Build history of the part. All positions in model axes, mm. Face numbers are marked on the shaded views. A direction names the side the tool comes from. Round coordinates to 2 decimals unless told otherwise and drop trailing zeros. Write each loop counter-clockwise with the first axis right and the second up, starting at its lowest first coordinate (ties: lowest second). Pieces come first, ordered by that corner, then holes.
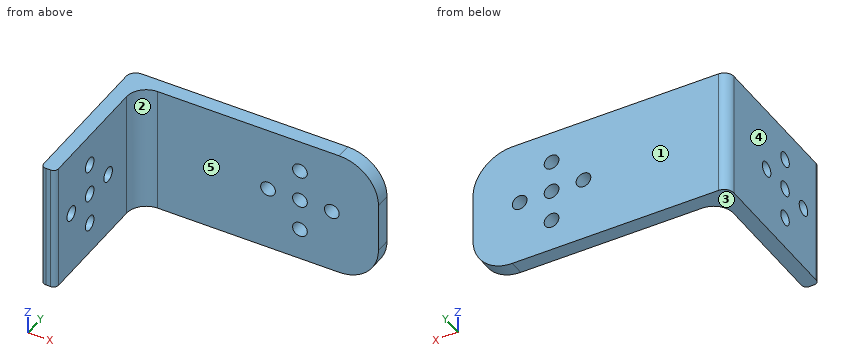
Autodesk Inventor part; units mm, degrees
ref_plane "YZ Plane" through (0, 0, 0) normal (1, 0, 0) x (0, 1, 0)
ref_plane "XZ Plane" through (0, 0, 0) normal (0, 1, 0) x (-1, 0, 0)
ref_plane "XY Plane" through (0, 0, 0) normal (0, 0, 1) x (1, 0, 0)
sketch "Sketch1" plane through (0, 0, 0) normal (0, 0, 1) x (1, 0, 0)
  line L0 (0, 0) -> (-49, 0)
  line L1 (-49, 0) -> (-49, 18)
  line L2 (-49, 18) -> (0, 18) construction
  line L3 (-49, 18) -> (-52, 18)
  line L4 (-52, 18) -> (-52, -3)
  line L5 (-52, -3) -> (0, -3)
  line L6 (0, -3) -> (0, 0)
  dimension "d0" = 18
  dimension "d1" = 3
  dimension "d2" = 3
  dimension "d3" = 52
extrude "Extrusion1" add sketch "Sketch1" along normal blind 10
mirror "Mirror1" about plane through (-32.0411, 1.4589, 0) normal (0, 0, -1) of "Extrusion1"
mirror "Mirror2" about plane through (-49, 18, 0) normal (0, 1, 0) of "Extrusion1", "Mirror1"
sketch "Sketch4" plane through (0, -3, -10) normal (0, 0, -1) x (-1, 0, 0)
  line L0 (0, 3) -> (49, 3)
  line L1 (0, 0) -> (0, 3)
  line L2 (52, 0) -> (0, 0)
  line L3 (52, 42) -> (52, 0)
  line L4 (52, 42) -> (0, 42)
  line L5 (0, 42) -> (0, 39)
  line L6 (0, 39) -> (49, 39)
  line L7 (49, 39) -> (49, 3)
  line L8 (0, 3) -> (49, 3)
  line L9 (0, 0) -> (0, 3)
  line L10 (52, 0) -> (0, 0)
  line L11 (52, 42) -> (52, 0)
  line L12 (52, 42) -> (0, 42)
  line L13 (0, 42) -> (0, 39)
  line L14 (0, 39) -> (49, 39)
  line L15 (49, 39) -> (49, 3)
extrude "Extrusion4" add sketch "Sketch4" along normal blind 5
mirror "Mirror3" about plane through (0, 0, 0) normal (0, 0, 1) of "Extrusion4"
sketch "Sketch11" plane through (-52, -3, -15) normal (0, -1, 0) x (1, 0, 0)
  line L0 (52, 0) -> (52, 30)
  line L1 (52, 30) -> (0, 30)
  line L2 (0, 0) -> (0, 30)
  line L3 (52, 0) -> (0, 0)
  line L4 (52, 0) -> (52, 30)
  line L5 (52, 30) -> (0, 30)
  line L6 (0, 0) -> (0, 30)
  line L7 (52, 0) -> (0, 0)
  point P0 (52, 15)
extrude "Extrusion11" cut sketch "Sketch11" against normal blind 10
sketch "Sketch13" plane through (0, 36, -15) normal (1, 0, 0) x (0, 0, -1)
  line L0 (-30, 3) -> (-28, 3)
  line L1 (-28, 3) -> (-28, -29)
  line L2 (-28, -29) -> (-30, -29)
  line L3 (-30, -29) -> (-30, 3)
  line L4 (-30, -29) -> (0, -29)
  point P0 (-15, -36)
  dimension "d65" = 2
extrude "Extrusion13" cut sketch "Sketch13" against normal up to next
mirror "Mirror4" about plane through (0, 0, 0) normal (0, 0, 1) of "Extrusion13"
sketch "Sketch14" plane through (-52, 7, 13) normal (-1, 0, 0) x (0, 0, 1)
  line L0 (-26, 32) -> (-26, 0)
  line L1 (-26, 0) -> (0, 0)
  line L2 (0, 32) -> (-26, 32)
  circle A0 centre (-13, 12) radius 6.5 construction
  line L3 (-13, 12) -> (-26, 12) construction
  line L4 (-13, 12) -> (-13, 32) construction
  circle A1 centre (-13, 12) radius 1.5
  circle A2 centre (-13, 18.5) radius 1.5
  point P0 (-13, -7)
  point P1 (-13, 0)
  dimension "d68" = 13
  dimension "d69" = 20
  dimension "d71" = 3
  dimension "d72" = 3
extrude "Extrusion14" cut sketch "Sketch14" against normal up to next
pattern_circular "Circular Pattern6" count 4 over 360 about axis through (-52, 19, 0) along (1, 0, 0) of "Extrusion14"
sketch "Sketch15" plane through (-49, 36, 13) normal (0, -1, 0) x (1, 0, 0)
  line L0 (49, -26) -> (49, 0)
  line L1 (49, 0) -> (0, 0)
  circle A0 centre (33, -13) radius 6.5 construction
  line L2 (33, -13) -> (33, 0) construction
  circle A1 centre (33, -6.5) radius 1.5
  circle A2 centre (33, -13) radius 1.5
  point P0 (49, -13)
  point P1 (49, -13)
  dimension "d78" = 13
  dimension "d79" = 16
  dimension "d80" = 3
  dimension "d81" = 3
extrude "Extrusion15" cut sketch "Sketch15" against normal up to next
pattern_circular "Circular Pattern7" count 4 over 360 about axis through (-16, 36, 0) along (0, 1, 0) of "Extrusion15"
fillet "Fillet1" radius 8 2 edges at (0, 37.5, -13) (0, 37.5, 13)
sketch "Sketch18" plane through (-52, 39, 13) normal (0, 1, 0) x (1, 0, 0)
  arc A0 (44, 0) -> (52, 8) centre (44, 8) ccw
  line L0 (52, 8) -> (52, 18)
  arc A1 (52, 18) -> (44, 26) centre (44, 18) ccw
  line L1 (44, 26) -> (0, 26)
  line L2 (0, 0) -> (0, 26)
  line L3 (0, 0) -> (44, 0)
  circle A2 centre (36, 13) radius 1.5
  circle A3 centre (36, 6.5) radius 1.5
  circle A4 centre (29.5, 13) radius 1.5
  circle A5 centre (42.5, 13) radius 1.5
  circle A6 centre (36, 19.5) radius 1.5
  point P0 (52, 13)
  dimension "d93" = 26
fillet "Fillet2" radius 4 1 edges at (-49, 36, 0)
fillet "Fillet3" radius 2 1 edges at (-52, 39, 0)
fillet "Fillet4" radius 1 2 edges at (-49, 7, 0) (-52, 7, 0)
equation "\"d72\" = d71"
properties part number "L_micro_sergei_dines"
1) Pin check, flat tips, straight feed: pin 1 Ø2.5 at (y, z) = (25.5, 0) entering from -X; pin 2 Ø3.5 at (y, z) = (12.5, 0) entering from -X; pin 3 Ø8 at (x, z) = (-22, 5.5) entering from -Y; pin 4 Ø12 at (y, z) = (20, 2.5) entering from +X. Stop position of each tip, or through.
Results:
pin 1: passes through
pin 2: stops at x = -52
pin 3: stops at y = 36
pin 4: stops at x = -49
2) Which spindle directions (+Z, -Z, +X, -X, +Y, -Y) get a long thin tool onto all of the face, cutting with end or side? Do the marked faces 4 and 5. Say none if no direction does.
Results:
face 4: +Z, -Z, -X, +Y, -Y
face 5: +Z, -Z, +X, -Y
3) Wall check: L1, parallel to Y at x = -14.5, z = 1.5; L2, parallel to X at y = 13, z = 6; L3, parallel to Z at x = -22.5, y = 37.9. Give the ranges that are in metal, low to high.
Results:
L1: y = 36 to 39
L2: x = -52 to -49
L3: z = -13 to -1.5, 1.5 to 13
4) Slice it at A-A (y = 19). Write the cut outline in (x, z).
Results:
outline: (-52, -13) - (-49, -13) - (-49, -8) - (-52, -8) - close; (-52, -5) - (-49, -5) - (-49, -1.5) - (-52, -1.5) - close; (-52, 1.5) - (-49, 1.5) - (-49, 5) - (-52, 5) - close; (-52, 8) - (-49, 8) - (-49, 13) - (-52, 13) - close
5) Mould opens along Y. For the marked faces 1, 2 and 3 say: released by +Y, released by -Y, zero draft, split by the parting line, or undercut.
Results:
face 1: released by +Y
face 2: released by -Y
face 3: zero draft
6) Slice it at D-D (y = 25.5). Write the cut outline in (x, z), plus the area to 3 significant figures.
Results:
outline: (-52, -13) - (-49, -13) - (-49, -1.5) - (-52, -1.5) - close; (-52, 1.5) - (-49, 1.5) - (-49, 13) - (-52, 13) - close
area: 69.0 mm2
7) Slice it at C-C (x = -22.5). Write the cut outline in (y, z), plus the area to 3 significant figures.
Results:
outline: (36, -13) - (39, -13) - (39, -1.5) - (36, -1.5) - close; (36, 1.5) - (39, 1.5) - (39, 13) - (36, 13) - close
area: 69.0 mm2
8) Slice it at B-B (z = 0). Count the separate pieces of the cut face and the enclosed holes in it, plus the area to 3 significant figures.
Results:
separate pieces: 7
enclosed holes: 0
area: 191 mm2
